CAD build for the part. Positions are in the model's coordinates, mm. A direction names the side the tool comes from. Round coordinates to 2 decimals unless told otherwise and drop trailing zeros. Loops run counter-clockwise (first coordinate to the right, second up) from the corner with the lowest first, then second, coordinate; pieces in that order, holes last. Notation, with made-up numbers: (62, -22.5) -> (95, -22.5) arc R6 ccw to (95, -11.5) -> close; hole circle Ø1 at (21, 81.5). An arc over 180 degrees is marked (long way). Answer as CSV lines item,"result".
Autodesk Inventor part; units mm, degrees
ref_plane "YZ Plane" through (0, 0, 0) normal (1, 0, 0) x (0, 1, 0)
ref_plane "XZ Plane" through (0, 0, 0) normal (0, 1, 0) x (-1, 0, 0)
ref_plane "XY Plane" through (0, 0, 0) normal (0, 0, 1) x (1, 0, 0)
sketch "Sketch1" plane through (0, 0, 0) normal (0, 0, 1) x (1, 0, 0)
  line L0 (0, 0) -> (457.2, 0)
  line L1 (457.2, 0) -> (457.2, 28.58)
  line L2 (457.2, 28.58) -> (72.12, 28.58)
  line L3 (0, 28.58) -> (0, 0)
  line L4 (0, 8.7151) -> (0, 28.58)
  line L5 (72.12, 28.58) -> (72.12, 57.5527)
  line L6 (72.12, 57.5527) -> (0, 57.5527)
  line L7 (0, 57.5527) -> (0, 28.58)
  dimension "d0" = 457.2
  dimension "d2" = 28.58
  dimension "d4" = 72.12
extrude "Extrusion1" add sketch "Sketch1" along normal blind 12.7
sketch "Sketch2" plane through (72.12, 28.58, 0) normal (1, 0, 0) x (0, 0, -1)
  circle A0 centre (-6.0784, 15.0544) radius 4.7759
  line L0 (0, 28.9727) -> (-12.7, 28.9727)
  line L1 (-12.7, 0) -> (-12.7, 28.9727)
  point P0 (0, -28.58)
extrude "Extrusion2" add sketch "Sketch2" along normal blind 396.0622
sketch "Sketch3" plane through (72.12, 28.58, 0) normal (0, 1, 0) x (1, 0, 0)
  point P0 (-72.12, 0)
sketch "Sketch4" plane through (0, 0, 12.7) normal (0, 0, 1) x (1, 0, 0)
  circle A0 centre (12.7, 12.7) radius 6.35
  line L0 (0, 0) -> (457.2, 0)
  line L1 (0, 57.5527) -> (0, 0)
  dimension "d12" = 12.7
  dimension "d13" = 12.7
  dimension "d14" = 12.7
hole "Hole1" at (12.7, 12.7, 12.7) direction (0, 0, -1) diameter 12.7 end through all
equation "\"d20\" = Thickness"
equation "\"BendRadius\" = Thickness"
equation "\"BendReliefWidth\" = Thickness"
equation "\"BendReliefDepth\" = 0.5 * Thickness"
equation "\"CornerReliefSize\" = 4 * Thickness"
equation "\"MinimumRemnant\" = 2 * Thickness"
equation "\"TransitionRadius\" = BendRadius"
equation "\"JacobiRadiusSize\" = BendRadius"
equation "\"GapSize\" = Thickness"
properties part number "new bolt"
Q1. Slice it at C-C, the plane z = 6. Give the cut face in (x, y), and give its area (3 significant figures).
Results:
outline,"(0, 0) -> (457.2, 0) -> (457.2, 28.58) -> (72.12, 28.58) -> (72.12, 38.86) -> (468.18, 38.86) -> (468.18, 48.41) -> (72.12, 48.41) -> (72.12, 57.55) -> (0, 57.55) -> close; hole circle Ø12.7 at (12.7, 12.7)"
area,"18,800 mm2"
Q2. Drop flat-ended pins along their axis: pin 1 Ø1.5 at (x, z) = (193, 4) entering from +Y; pin 2 Ø4 at (y, z) = (18, 8) entering from +X; pin 3 Ø1.5 at (x, z) = (199.5, 7.5) entering from +Y. Give the stop position or say it passes through.
Results:
pin 1,"y = 48.22"
pin 2,"x = 457.2"
pin 3,"y = 48.36"
Q3. Slice it at D-D, the plane x = 348. Give the cut face in (y, z), and give its area (3 significant figures).
Results:
outline,"(0, 0) -> (28.58, 0) -> (28.58, 12.7) -> (0, 12.7) -> close; circle Ø9.55 at (43.63, 6.08)"
area,"435 mm2"
Q4. Probe L1, parallel to Y at x = 12.7, z = 5; L2, parallel to X at y = 12.7, z = 5; L3, parallel to Y at x = 140.5, z = 4. List the from-to ranges inside material, lowest first. Write a range as [from, to].
Results:
L1,"[0, 6.35], [19.05, 57.55]"
L2,"[0, 6.35], [19.05, 457.2]"
L3,"[0, 28.58], [39.33, 47.93]"
Q5. Slice it at B-B, the plane x = 12.7. Give the cut face in (y, z), and give its area (3 significant figures).
Results:
outline,"(0, 0) -> (6.35, 0) -> (6.35, 12.7) -> (0, 12.7) -> close; (19.05, 0) -> (57.55, 0) -> (57.55, 12.7) -> (19.05, 12.7) -> close"
area,"570 mm2"
Q6. Tool access for faces 1 (the cylindrical face through (267.4, 48.3, 7.1)), 2 (the flat face through (267, 28.58, 6)), 3 (the flat face through (457.2, 14, 6)), 4 (the flat face through (225, 16, 12.7)): list every direction of +Z, -Z, +X, -X, +Y, -Y with a clear straight run to the whole face (end or side of a thin tool).
Results:
face 1,"+X"
face 2,"+Z, -Z, +X"
face 3,"+Z, -Z, +X, -Y"
face 4,"+Z, +X, -X, +Y, -Y"
Q7. Two-plate mould, pull along Y, no slides. Class faces 5 (the flat face through (72.12, 39.6, 9.1)), 6 (the flat face through (37, 57.553, 6)), 7 (the flat face through (468.182, 44, 6)): pulls with the +Y half, pulls with the -Y half, needs draft (parallel to the pull), parting line crosses it, or undercut.
Results:
face 5,"undercut"
face 6,"pulls with the +Y half"
face 7,"needs draft"
Q8. Slice it at A-A, the plane y = 12.7. Give the cut face in (x, z), and give its area (3 significant figures).
Results:
outline,"(0, 0) -> (6.35, 0) -> (6.35, 12.7) -> (0, 12.7) -> close; (19.05, 0) -> (457.2, 0) -> (457.2, 12.7) -> (19.05, 12.7) -> close"
area,"5,650 mm2"
